The model under review builds one solid part; all positions refer to its coordinate system, in mm. Round coordinates to 2 decimals unless told otherwise and drop trailing zeros. Order: outer loops, then holes, each group sorted by start corner. A loop starts at its lowest first (then second) coordinate and runs counter-clockwise, first axis right, second up. Notation, with made-up numbers: M 21.25,55.5 L 76.25,55.5 A18 ccw 76.25,63.5 Z; hole C -6.75,71.25 d6. An arc over 180 degrees is marked long. Answer as a JSON object with one key per item and string values. Group by question number.
1. Clearance check with flat-ended pins moving along their axes: P1, Ø6, axis at x = 3.5, y = 17, coming from the -Z side; P2, Ø8, axis at x = -14.5, y = 39.5, coming from the +Z side; P3, Ø4, axis at y = 55, z = -10.5, coming from the +X side. State where each tip first meets the part, or that it passes through.
2. Add section A-A on y = 24.5. State the section outline as (x, z) points, and give its area (3 significant figures).
3. To check wall thickness, follow probe 1 along X at (y, z) = (46.25, 0); probe 2 along Z at (x, y) = (0, 13.9). State the ranges of each line that lie inside material, in increasing order. Write a range as [from, to].
Autodesk Inventor part; units mm, degrees
ref_plane "YZ Plane" through (0, 0, 0) normal (1, 0, 0) x (0, 1, 0)
ref_plane "XZ Plane" through (0, 0, 0) normal (0, 1, 0) x (-1, 0, 0)
ref_plane "XY Plane" through (0, 0, 0) normal (0, 0, 1) x (1, 0, 0)
sketch "Sketch2" plane through (0, 0, 0) normal (0, 0, 1) x (1, 0, 0)
  line L0 (0, 0) -> (20.75, 0)
  line L1 (0, 3.5) -> (18.25, 3.5)
  line L2 (20.75, 1.25) -> (20.75, 0)
  line L3 (0, 0) -> (0, 3.5)
  line L4 (18.25, 3.5) -> (18.25, 2.1599)
  line L5 (17.25, 3.5) -> (17.25, 1.4597)
  line L6 (19.75, 0) -> (19.75, 0.5498)
  line L7 (19.75, 0.5498) -> (17.25, 1.4597)
  line L8 (20.75, 1.25) -> (18.25, 2.1599)
  dimension "d4" = 1.25
  dimension "d6" = 36.5
  dimension "d7" = 41.5
  dimension "d9" = 34.5
  dimension "d10" = 1
  dimension "d12" = 1
  dimension "d15" = 110
  dimension "d16" = 1
  dimension "d17" = 2.25
revolve "Revolution1" add sketch "Sketch2" angle 360 about axis through (0, 0, 0) along (0, 1, 0) contours L6 L7 L5 L1 L4 L8 L2 L0
mirror "Mirror1" about plane through (17.25, 3.5, 0) normal (0, 1, 0) of "Revolution1"
pattern_linear "Rectangular Pattern1" count 10 spacing 7 along (0, 1, 0) of "Revolution1", "Mirror1"
equation "\"d12\" = d10"
equation "\"d16\" = d10"
properties part number "40mm Vacuum Hose" material "PVC, Unplasticized"
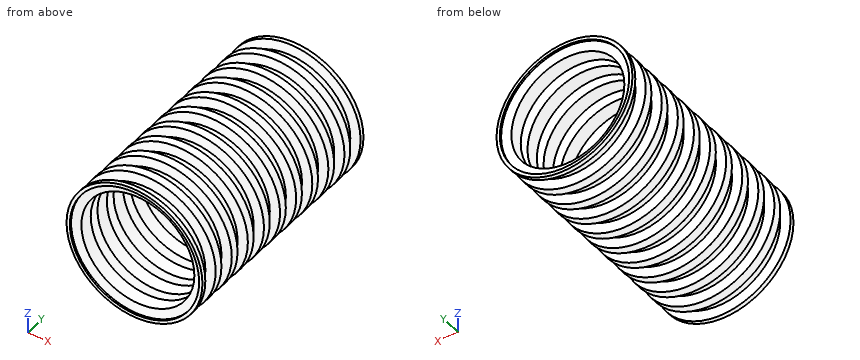
Recorded:
{
 "1": {"P1": "stops at z = -20.72", "P2": "stops at z = 17.78", "P3": "stops at x = 18.93"},
 "2": {"outline": "C 0,0 d36.5; hole C 0,0 d34.5", "area": "112 mm²"},
 "3": {"probe 1": "x = [-18.25, -17.25], [17.25, 18.25]", "probe 2": "z = [-20.75, -19.75], [19.75, 20.75]"}
}
